Check sheet for the modelled part. Datum: model origin and axes. Units: mm. A direction names the side the tool comes from. Round coordinates to 2 decimals unless told otherwise and drop trailing zeros. Loops run counter-clockwise (first coordinate to the right, second up) from the corner with the lowest first, then second, coordinate; pieces in that order, holes last. Notation, with made-up numbers: (65, 28.25) -> (106, 28.25) arc R4 ccw to (106, 34.25) -> close; hole circle Ø3 at (-22.5, -15.75). An arc over 180 degrees is marked (long way). Return JSON: item names as keys, results as strings.
from build123d import *

# Parameters (mm, degrees)
SKETCH1_W           = 114.3
SKETCH1_H           = 88.9
BOSS_EXTRUDE1_DEPTH = 35.56
SHELL1_T            = -2.54
FILLET1_R           = 2.54
SKETCH2_R           = 2.54
BOSS_EXTRUDE2_DEPTH = 33.02
SKETCH4_W           = 13.97
SKETCH4_H           = 10.541
CUT_EXTRUDE2_DEPTH  = 0.9525
SKETCH5_R           = 2.54
BOSS_EXTRUDE3_DEPTH = 3.175
SKETCH6_R           = 0.9525
BOSS_EXTRUDE4_DEPTH = 2.54
CUT_EXTRUDE3_REACH  = 129.69
SKETCH7_W           = 10.16
SKETCH7_H           = 13.462
SKETCH8_W           = 16.51
SKETCH8_H           = 19.812
SKETCH8_W_2         = 10.16
SKETCH8_H_2         = 13.462
BOSS_EXTRUDE5_DEPTH = 3.175
CHAMFER1_SIZE       = 2.54
FILLET2_R           = 3.175


with BuildPart() as part:
    # Sketch1 → Boss-Extrude1 (new body)
    with BuildSketch(Plane(origin=(0, 0, 0), x_dir=(1, 0, 0), z_dir=(0, 1, 0))):
        Rectangle(SKETCH1_W, SKETCH1_H)
    extrude(amount=BOSS_EXTRUDE1_DEPTH)

    # Shell1
    shell1_openings = [part.faces().sort_by_distance(p)[0] for p in [
        (0, 35.56, 0),
    ]]
    offset(amount=SHELL1_T, openings=shell1_openings, kind=Kind.INTERSECTION)

    # Fillet1
    fillet1_edges = [part.edges().sort_by_distance(p)[0] for p in [
        (-54.61, 19.05, -41.91),
        (-54.61, 19.05, 41.91),
        (54.61, 19.05, 41.91),
        (54.61, 19.05, -41.91),
        (-57.15, 17.78, -44.45),
        (57.15, 17.78, -44.45),
        (57.15, 17.78, 44.45),
        (-57.15, 17.78, 44.45),
    ]]
    fillet(fillet1_edges, radius=FILLET1_R)

    # Sketch2 → Boss-Extrude2 (add)
    with BuildSketch(Plane(origin=(0, 35.56, 0), x_dir=(1, 0, 0), z_dir=(0, 1, 0))):
        with Locations((-54.61, 41.91)):
            Circle(SKETCH2_R)
        with Locations((54.61, 41.91)):
            Circle(SKETCH2_R)
        with Locations((54.61, -41.91)):
            Circle(SKETCH2_R)
        with Locations((-54.61, -41.91)):
            Circle(SKETCH2_R)
    extrude(amount=-BOSS_EXTRUDE2_DEPTH)

    # Sketch4 → Cut-Extrude2 (cut)
    with BuildSketch(Plane.ZY.offset(-54.61)):
        with Locations((15.875, 7.8105)):
            Rectangle(SKETCH4_W, SKETCH4_H)
    extrude(amount=-CUT_EXTRUDE2_DEPTH, mode=Mode.SUBTRACT)

    # Sketch5 → Boss-Extrude3 (add)
    with BuildSketch(Plane(origin=(0, 2.54, 0), x_dir=(1, 0, 0), z_dir=(0, 1, 0))):
        with Locations(Location((24.892, 0, 0), (0, 0, 90))):
            Circle(SKETCH5_R)
        with Locations(Location((50.292, 0, 0), (0, 0, 90))):
            Circle(SKETCH5_R)
        with Locations(Location((24.892, -35.56, 0), (0, 0, 90))):
            Circle(SKETCH5_R)
        with Locations(Location((50.292, -35.56, 0), (0, 0, 90))):
            Circle(SKETCH5_R)
    extrude(amount=BOSS_EXTRUDE3_DEPTH)

    # Sketch6 → Boss-Extrude4 (add)
    with BuildSketch(Plane(origin=(0, 5.715, 0), x_dir=(1, 0, 0), z_dir=(0, 1, 0))):
        with Locations(Location((24.892, 0, 0), (0, 0, 270))):
            Circle(SKETCH6_R)
        with Locations(Location((50.292, 0, 0), (0, 0, 270))):
            Circle(SKETCH6_R)
        with Locations(Location((50.292, -35.56, 0), (0, 0, 270))):
            Circle(SKETCH6_R)
        with Locations(Location((24.892, -35.56, 0), (0, 0, 270))):
            Circle(SKETCH6_R)
    extrude(amount=BOSS_EXTRUDE4_DEPTH)

    # Sketch7 → Cut-Extrude3 (cut, up to next)
    with BuildSketch(Plane(origin=(57.15, 0, 0), x_dir=(0, 0, -1), z_dir=(1, 0, 0)), mode=Mode.PRIVATE) as cut_extrude3_sk1:
        with Locations((-27.305, 13.335)):
            Rectangle(SKETCH7_W, SKETCH7_H)
    cut_extrude3_tool1 = extrude(cut_extrude3_sk1.sketch, amount=-CUT_EXTRUDE3_REACH, mode=Mode.PRIVATE) & part.part
    add(cut_extrude3_tool1.solids().sort_by_distance((57.15, 13.335, 27.305))[0], mode=Mode.SUBTRACT)

    # Sketch8 → Boss-Extrude5 (add)
    with BuildSketch(Plane(origin=(57.15, 0, 0), x_dir=(0, 0, -1), z_dir=(1, 0, 0))):
        with Locations((-27.305, 13.335)):
            Rectangle(SKETCH8_W, SKETCH8_H)
        with Locations((-27.305, 13.335)):
            Rectangle(SKETCH8_W_2, SKETCH8_H_2, mode=Mode.SUBTRACT)
    extrude(amount=BOSS_EXTRUDE5_DEPTH)

    # Chamfer1
    chamfer1_edges = [part.edges().sort_by_distance(p)[0] for p in [
        (60.325, 13.335, 32.385),
        (60.325, 6.604, 27.305),
        (60.325, 13.335, 22.225),
        (60.325, 20.066, 27.305),
    ]]
    chamfer(chamfer1_edges, length=CHAMFER1_SIZE)

    # Fillet2
    fillet2_edges = [part.edges().sort_by_distance(p)[0] for p in [
        (57.15, 3.429, 27.305),
        (57.15, 13.335, 19.05),
        (57.15, 23.241, 27.305),
        (57.15, 13.335, 35.56),
    ]]
    fillet(fillet2_edges, radius=FILLET2_R - 0.0001)  # a hair under: the kernel refuses the full size


solid = part.part
Q1. Section check B-B (x = 11.5). Record the boundary of the cut face in (y, z).
Results list:
{"outline": "(0, -44.45) -> (35.56, -44.45) -> (35.56, -41.91) -> (2.54, -41.91) -> (2.54, 41.91) -> (35.56, 41.91) -> (35.56, 44.45) -> (0, 44.45) -> close"}
Q2. Draft check along Z on faces 4 (the flat face through (-1, 18, 44.45)), 5 (the flat face through (59.04, 5.35, 27.41)), 6 (the cylindrical face through (58.1, 24.15, 27.14)). Enter one of: released by +Z, released by -Z, zero draft, split by the parting line, or undercut.
Results list:
{"face 4": "released by +Z", "face 5": "undercut", "face 6": "zero draft"}
Q3. Section check A-A (y = 31.5). Record the boundary of the cut face in (x, z), then the cut area to 3 significant figures.
Results list:
{"outline": "(-57.15, -41.91) arc R2.54 ccw to (-54.61, -44.45) -> (54.61, -44.45) arc R2.54 ccw to (57.15, -41.91) -> (57.15, 41.91) arc R2.54 ccw to (54.61, 44.45) -> (-54.61, 44.45) arc R2.54 ccw to (-57.15, 41.91) -> close; hole (-54.61, -39.37) arc R2.54 cw to (-52.07, -41.91) -> (52.07, -41.91) arc R2.54 cw to (54.61, -39.37) -> (54.61, 39.37) arc R2.54 cw to (52.07, 41.91) -> (-52.07, 41.91) arc R2.54 cw to (-54.61, 39.37) -> close", "area": "1,020 mm^2"}
Q4. Material ranges on line 1 (X direction, y = 15, z = 4); line 2 (Z direction, x = -20, y = 25); line 3 (Y direction, x = 43.5, z = -3.5), recorded low to high.
Results list:
{"line 1": "-57.15 to -54.61, 54.61 to 57.15", "line 2": "-44.45 to -41.91, 41.91 to 44.45", "line 3": "0 to 2.54"}
Q5. Tool access check on faces 1 (the flat face through (26, 5.715, 0)), 2 (the flat face through (60.325, 13.4, 35.3)), 3 (the flat face through (59, 13.2, 33.6)). Record the directions out of +Z, -Z, +X, -X, +Y, -Y that give a thin tool (end or side, any length) a straight path to the whole face; none if there is none.
Results list:
{"face 1": "+Y", "face 2": "+Z, -Z, +X, +Y, -Y", "face 3": "+X"}
Q6. Go/stop test with flat-tipped pins: pin 1 (1.5 mm diameter, centred on x = 25.5, z = -1, fed in from +Y) (3 decimals); pin 2 (8 mm diameter, centred on x = 20.5, z = 13, fed in from +Y); pin 3 (0.8 mm diameter, centred on x = 55, y = 4, fed in from -Z); pin 4 (2 mm diameter, centred on y = 32, z = 10.5, fed in from +X). Record where each tip stops, or that it passes through.
Results list:
{"pin 1": "y = 8.255", "pin 2": "y = 2.54", "pin 3": "z = -44.45", "pin 4": "x = 57.15"}
Q7. Section check C-C (z = 4.5). Record the boundary of the cut face in (x, y), then the cut area to 3 significant figures.
Results list:
{"outline": "(-57.15, 0) -> (57.15, 0) -> (57.15, 35.56) -> (54.61, 35.56) -> (54.61, 2.54) -> (-54.61, 2.54) -> (-54.61, 35.56) -> (-57.15, 35.56) -> close", "area": "458 mm^2"}
